from build123d import *

# Parameters (mm, degrees)
P_IDAT_VYSUNUT_M1_DEPTH  = 5
SKICA2_R                 = 2
ODEBRAT_VYSUNUT_M1_DEPTH = 148.885090526
SKICA4_R                 = 6
ODEBRAT_VYSUNUT_M3_DEPTH = 10
SKICA5_R                 = 3
ODEBRAT_VYSUNUT_M4_DEPTH = 2
SKICA6_R                 = 12
SKICA6_R_2               = 8.5
SKICA6_R_3               = 7.5
ODEBRAT_VYSUNUT_M5_DEPTH = 148.885090526


with BuildPart() as part:
    # Skica1 → Přidat vysunutím1 (new body)
    with BuildSketch(Plane.XY):
        Polygon((-103, 106), (103, 106), (103, 103), (101, 103), (101, -103), (103, -103), (103, -106), (-103, -106), (-103, -103), (-101, -103), (-101, 103), (-103, 103), align=None)
    extrude(amount=P_IDAT_VYSUNUT_M1_DEPTH)

    # Skica2 → Odebrat vysunutím1 (cut, through all)
    with BuildSketch(Plane.XY.offset(5)):
        with Locations((-85, 101)):
            Circle(SKICA2_R)
        with Locations((0, 101)):
            Circle(SKICA2_R)
        with Locations((85, 101)):
            Circle(SKICA2_R)
        with Locations(Location((-85, -101, 0), (0, 0, 180))):
            Circle(SKICA2_R)
        with Locations(Location((0, -101, 0), (0, 0, 180))):
            Circle(SKICA2_R)
        with Locations(Location((85, -101, 0), (0, 0, 180))):
            Circle(SKICA2_R)
    extrude(amount=-ODEBRAT_VYSUNUT_M1_DEPTH, mode=Mode.SUBTRACT)

    # Skica4 → Odebrat vysunutím3 (cut)
    with BuildSketch(Plane.XY.offset(5)):
        with Locations((48, 48)):
            Circle(SKICA4_R)
        with Locations(Location((-48, 48, 0), (0, 0, 180))):
            Circle(SKICA4_R)
        with Locations(Location((48, -48, 0), (0, 0, 180))):
            Circle(SKICA4_R)
        with Locations((-48, -48)):
            Circle(SKICA4_R)
        with BuildLine():
            Line((40.918682945, 58.939196308), (16.459341473, 83.469598154))
            ThreePointArc((16.459341473, 83.469598154), (15.381991272, 88.916766909), (20, 92))
            Line((20, 92), (76, 92))
            ThreePointArc((76, 92), (80.618008728, 88.916766909), (79.540658527, 83.469598154))
            Line((79.540658527, 83.469598154), (55.081317055, 58.939196308))
            ThreePointArc((55.081317055, 58.939196308), (48, 56), (40.918682945, 58.939196308))
        make_face()
        with BuildLine():
            Line((37.060803692, 55.081317055), (12.530401846, 79.540658527))
            ThreePointArc((12.530401846, 79.540658527), (7.083233091, 80.618008728), (4, 76))
            Line((4, 76), (4, 20))
            ThreePointArc((4, 20), (7.083233091, 15.381991272), (12.530401846, 16.459341473))
            Line((12.530401846, 16.459341473), (37.060803692, 40.918682945))
            ThreePointArc((37.060803692, 40.918682945), (40, 48), (37.060803692, 55.081317055))
        make_face()
        with BuildLine():
            Line((58.939196308, 40.918682945), (83.469598154, 16.459341473))
            ThreePointArc((83.469598154, 16.459341473), (88.916766909, 15.381991272), (92, 20))
            Line((92, 20), (92, 76))
            ThreePointArc((92, 76), (88.916766909, 80.618008728), (83.469598154, 79.540658527))
            Line((83.469598154, 79.540658527), (58.939196308, 55.081317055))
            ThreePointArc((58.939196308, 55.081317055), (56, 48), (58.939196308, 40.918682945))
        make_face()
        with BuildLine():
            Line((40.918682945, 37.060803692), (16.459341473, 12.530401846))
            ThreePointArc((16.459341473, 12.530401846), (15.381991272, 7.083233091), (20, 4))
            Line((20, 4), (76, 4))
            ThreePointArc((76, 4), (80.618008728, 7.083233091), (79.540658527, 12.530401846))
            Line((79.540658527, 12.530401846), (55.081317055, 37.060803692))
            ThreePointArc((55.081317055, 37.060803692), (48, 40), (40.918682945, 37.060803692))
        make_face()
        with BuildLine():
            Line((-40.918682945, 58.939196308), (-16.459341473, 83.469598154))
            ThreePointArc((-16.459341473, 83.469598154), (-15.381991272, 88.916766909), (-20, 92))
            Line((-20, 92), (-76, 92))
            ThreePointArc((-76, 92), (-80.618008728, 88.916766909), (-79.540658527, 83.469598154))
            Line((-79.540658527, 83.469598154), (-55.081317055, 58.939196308))
            ThreePointArc((-55.081317055, 58.939196308), (-48, 56), (-40.918682945, 58.939196308))
        make_face()
        with BuildLine():
            Line((-58.939196308, 55.081317055), (-83.469598154, 79.540658527))
            ThreePointArc((-83.469598154, 79.540658527), (-88.916766909, 80.618008728), (-92, 76))
            Line((-92, 76), (-92, 20))
            ThreePointArc((-92, 20), (-88.916766909, 15.381991272), (-83.469598154, 16.459341473))
            Line((-83.469598154, 16.459341473), (-58.939196308, 40.918682945))
            ThreePointArc((-58.939196308, 40.918682945), (-56, 48), (-58.939196308, 55.081317055))
        make_face()
        with BuildLine():
            Line((-55.081317055, 37.060803692), (-79.540658527, 12.530401846))
            ThreePointArc((-79.540658527, 12.530401846), (-80.618008728, 7.083233091), (-76, 4))
            Line((-76, 4), (-20, 4))
            ThreePointArc((-20, 4), (-15.381991272, 7.083233091), (-16.459341473, 12.530401846))
            Line((-16.459341473, 12.530401846), (-40.918682945, 37.060803692))
            ThreePointArc((-40.918682945, 37.060803692), (-48, 40), (-55.081317055, 37.060803692))
        make_face()
        with BuildLine():
            Line((-37.060803692, 40.918682945), (-12.530401846, 16.459341473))
            ThreePointArc((-12.530401846, 16.459341473), (-7.083233091, 15.381991272), (-4, 20))
            Line((-4, 20), (-4, 76))
            ThreePointArc((-4, 76), (-7.083233091, 80.618008728), (-12.530401846, 79.540658527))
            Line((-12.530401846, 79.540658527), (-37.060803692, 55.081317055))
            ThreePointArc((-37.060803692, 55.081317055), (-40, 48), (-37.060803692, 40.918682945))
        make_face()
        with BuildLine():
            Line((40.918682945, -58.939196308), (16.459341473, -83.469598154))
            ThreePointArc((16.459341473, -83.469598154), (15.381991272, -88.916766909), (20, -92))
            Line((20, -92), (76, -92))
            ThreePointArc((76, -92), (80.618008728, -88.916766909), (79.540658527, -83.469598154))
            Line((79.540658527, -83.469598154), (55.081317055, -58.939196308))
            ThreePointArc((55.081317055, -58.939196308), (48, -56), (40.918682945, -58.939196308))
        make_face()
        with BuildLine():
            Line((58.939196308, -55.081317055), (83.469598154, -79.540658527))
            ThreePointArc((83.469598154, -79.540658527), (88.916766909, -80.618008728), (92, -76))
            Line((92, -76), (92, -20))
            ThreePointArc((92, -20), (88.916766909, -15.381991272), (83.469598154, -16.459341473))
            Line((83.469598154, -16.459341473), (58.939196308, -40.918682945))
            ThreePointArc((58.939196308, -40.918682945), (56, -48), (58.939196308, -55.081317055))
        make_face()
        with BuildLine():
            Line((55.081317055, -37.060803692), (79.540658527, -12.530401846))
            ThreePointArc((79.540658527, -12.530401846), (80.618008728, -7.083233091), (76, -4))
            Line((76, -4), (20, -4))
            ThreePointArc((20, -4), (15.381991272, -7.083233091), (16.459341473, -12.530401846))
            Line((16.459341473, -12.530401846), (40.918682945, -37.060803692))
            ThreePointArc((40.918682945, -37.060803692), (48, -40), (55.081317055, -37.060803692))
        make_face()
        with BuildLine():
            Line((37.060803692, -40.918682945), (12.530401846, -16.459341473))
            ThreePointArc((12.530401846, -16.459341473), (7.083233091, -15.381991272), (4, -20))
            Line((4, -20), (4, -76))
            ThreePointArc((4, -76), (7.083233091, -80.618008728), (12.530401846, -79.540658527))
            Line((12.530401846, -79.540658527), (37.060803692, -55.081317055))
            ThreePointArc((37.060803692, -55.081317055), (40, -48), (37.060803692, -40.918682945))
        make_face()
        with BuildLine():
            Line((-37.060803692, -55.081317055), (-12.530401846, -79.540658527))
            ThreePointArc((-12.530401846, -79.540658527), (-7.083233091, -80.618008728), (-4, -76))
            Line((-4, -76), (-4, -20))
            ThreePointArc((-4, -20), (-7.083233091, -15.381991272), (-12.530401846, -16.459341473))
            Line((-12.530401846, -16.459341473), (-37.060803692, -40.918682945))
            ThreePointArc((-37.060803692, -40.918682945), (-40, -48), (-37.060803692, -55.081317055))
        make_face()
        with BuildLine():
            Line((-55.081317055, -58.939196308), (-79.540658527, -83.469598154))
            ThreePointArc((-79.540658527, -83.469598154), (-80.618008728, -88.916766909), (-76, -92))
            Line((-76, -92), (-20, -92))
            ThreePointArc((-20, -92), (-15.381991272, -88.916766909), (-16.459341473, -83.469598154))
            Line((-16.459341473, -83.469598154), (-40.918682945, -58.939196308))
            ThreePointArc((-40.918682945, -58.939196308), (-48, -56), (-55.081317055, -58.939196308))
        make_face()
        with BuildLine():
            Line((-58.939196308, -40.918682945), (-83.469598154, -16.459341473))
            ThreePointArc((-83.469598154, -16.459341473), (-88.916766909, -15.381991272), (-92, -20))
            Line((-92, -20), (-92, -76))
            ThreePointArc((-92, -76), (-88.916766909, -80.618008728), (-83.469598154, -79.540658527))
            Line((-83.469598154, -79.540658527), (-58.939196308, -55.081317055))
            ThreePointArc((-58.939196308, -55.081317055), (-56, -48), (-58.939196308, -40.918682945))
        make_face()
        with BuildLine():
            Line((-40.918682945, -37.060803692), (-16.459341473, -12.530401846))
            ThreePointArc((-16.459341473, -12.530401846), (-15.381991272, -7.083233091), (-20, -4))
            Line((-20, -4), (-76, -4))
            ThreePointArc((-76, -4), (-80.618008728, -7.083233091), (-79.540658527, -12.530401846))
            Line((-79.540658527, -12.530401846), (-55.081317055, -37.060803692))
            ThreePointArc((-55.081317055, -37.060803692), (-48, -40), (-40.918682945, -37.060803692))
        make_face()
    extrude(amount=-ODEBRAT_VYSUNUT_M3_DEPTH, mode=Mode.SUBTRACT)

    # Skica5 → Odebrat vysunutím4 (cut)
    with BuildSketch(Plane.XY.offset(5)):
        with Locations((-85, 101)):
            Circle(SKICA5_R)
        with Locations((0, 101)):
            Circle(SKICA5_R)
        with Locations((85, 101)):
            Circle(SKICA5_R)
        with Locations(Location((-85, -101, 0), (0, 0, 180))):
            Circle(SKICA5_R)
        with Locations(Location((0, -101, 0), (0, 0, 180))):
            Circle(SKICA5_R)
        with Locations(Location((85, -101, 0), (0, 0, 180))):
            Circle(SKICA5_R)
    extrude(amount=-ODEBRAT_VYSUNUT_M4_DEPTH, mode=Mode.SUBTRACT)

    # Skica6 → Odebrat vysunutím5 (cut, through all)
    with BuildSketch(Plane.XY.offset(5)):
        Circle(SKICA6_R)
        with Locations((-90, 0)):
            Circle(SKICA6_R_2)
        with Locations(Location((90, 0, 0), (0, 0, 180))):
            Circle(SKICA6_R_2)
        with Locations((-90, 90)):
            Circle(SKICA6_R_3)
        with Locations((90, 90)):
            Circle(SKICA6_R_3)
        with Locations((90, -90)):
            Circle(SKICA6_R_3)
        with Locations((-90, -90)):
            Circle(SKICA6_R_3)
        with Locations((0, 88)):
            Circle(SKICA6_R_3)
        with Locations(Location((0, -88, 0), (0, 0, 180))):
            Circle(SKICA6_R_3)
    extrude(amount=-ODEBRAT_VYSUNUT_M5_DEPTH, mode=Mode.SUBTRACT)


solid = part.part
Here's how the part is built. I have some questions about the finished solid (model axes, mm). A direction names the side the tool comes from. Coordinates: 2 decimals unless noted, no trailing zeros. Write each loop counter-clockwise with the first axis right and the second up, starting at its lowest first coordinate (ties: lowest second). Pieces come first, ordered by that corner, then holes.
Item 1: I want a section at A-A on y = -64. Write out the boundary of the cut face in (x, z).
Item 2: Will these pins go through, and if not, where does the flat tip stop? pin 1 (4.5 mm diameter, centred on x = 0, y = 101, fed in from -Z); pin 2 (2 mm diameter, centred on y = 72.5, z = 2, fed in from +X); pin 3 (3.5 mm diameter, centred on x = -85, y = -101, fed in from +Z); pin 4 (3 mm diameter, centred on y = 2.5, z = 3.5, fed in from -X).
Item 3: On a 3-axis mill with a long thin cutter (end or side, diameter ignored), from which of +Z, -Z, +X, -X, +Y, -Y can I reach the whole of each face in a straight line? I mean faces 1 (the flat face through (2, 100, 3)), 2 (the flat face through (-48, 92, 3)). Say none if no direction works.
Item 4: I want a section at B-B on z = 1.1. Count the separate pieces of the cut face and the enclosed holes in it, and give its area (3 significant figures).
Item 5: If I drill on line 1 (Y direction, x = 0, z = 2.7); line 2 (X direction, y = -101, z = 0.85); line 3 (X direction, y = -88, z = 1.9), over which ranges is the centre line in solid material (lowest first)?
Item 6: I want a section at C-C on y = 23.5. Write out the boundary of the cut face in (x, z).
Findings below:
1. outline: (-101, 0) - (-92, 0) - (-92, 5) - (-101, 5) - close; (-67.88, 0) - (-60.13, 0) - (-60.13, 5) - (-67.88, 5) - close; (-35.87, 0) - (-28.12, 0) - (-28.12, 5) - (-35.87, 5) - close; (-4, 0) - (4, 0) - (4, 5) - (-4, 5) - close; (28.12, 0) - (35.87, 0) - (35.87, 5) - (28.12, 5) - close; (60.13, 0) - (67.88, 0) - (67.88, 5) - (60.13, 5) - close; (92, 0) - (101, 0) - (101, 5) - (92, 5) - close
2. pin 1: stops at z = 0
2. pin 2: stops at x = 101
2. pin 3: passes through
2. pin 4: stops at x = -101
3. face 1: +Z
3. face 2: +Z, -Z
4. separate pieces: 1
4. enclosed holes: 35
4. area: 16,000 mm2
5. line 1: y = -106 to -103, -99 to -95.5, -80.5 to -12, 12 to 80.5, 95.5 to 99, 103 to 106
5. line 2: x = -101 to -87, -83 to -2, 2 to 83, 87 to 101
5. line 3: x = -101 to -97.23, -82.77 to -80.9, -15.1 to -7.5, 7.5 to 15.1, 80.9 to 82.77, 97.23 to 101
6. outline: (-101, 0) - (-92, 0) - (-92, 5) - (-101, 5) - close; (-76.41, 0) - (-68.6, 0) - (-68.6, 5) - (-76.41, 5) - close; (-27.4, 0) - (-19.59, 0) - (-19.59, 5) - (-27.4, 5) - close; (-4, 0) - (4, 0) - (4, 5) - (-4, 5) - close; (19.59, 0) - (27.4, 0) - (27.4, 5) - (19.59, 5) - close; (68.6, 0) - (76.41, 0) - (76.41, 5) - (68.6, 5) - close; (92, 0) - (101, 0) - (101, 5) - (92, 5) - close
